The model under review builds one solid part; all positions refer to its coordinate system, in mm. Face numbers are marked on the shaded views. A direction names the side the tool comes from. Coordinates: 2 decimals unless noted, no trailing zeros. Write each loop counter-clockwise with the first axis right and the second up, starting at its lowest first coordinate (ties: lowest second). Pieces come first, ordered by that corner, then holes. Notation, with made-up numbers: (81.25, 25) - (131.25, 25) arc R26 cw to (131.25, 63) - close; hole circle Ø2 at (68, -30). An arc over 180 degrees is marked (long way). Put each result on its own line as item: value. Start each with the question number.
Item 1: For pin 1 (3 mm diameter, centred on x = -25.5, z = 3.5, fed in from +Y); pin 2 (5 mm diameter, centred on x = 12.5, z = 3, fed in from +Y); pin 3 (4 mm diameter, centred on x = -17, y = 5, fed in from +Z), all flat-tipped, find the tip position at first contact; note any pin that passes through.
Item 2: Consider section B-B on x = 3. Give the boundary of the cut face in (y, z), then the cut area to 3 significant figures.
Item 3: To check wall thickness, follow L1, parallel to Y at x = 7, z = 0; L2, parallel to X at y = -7.25, z = 4.5; L3, parallel to Y at x = 16, z = 0.75. State the ranges of each line that lie inside material, in increasing order. Write a range as [from, to].
Item 4: Machinability: for the marked faces 1 and 2, which of the approach directions +Z, -Z, +X, -X, +Y, -Y give a long, thin tool a straight path to every point of the face, cutting with its end or side? Answer none if there is none.
Item 5: Consider section C-C on x = 25.5. Give the boundary of the cut face in (y, z).
Item 6: Mouldability with a two-part tool opening along X and no side actions: class the marked faces 3, 4, 5 and 6 as pulls with the +X half, pulls with the -X half, needs draft (parallel to the pull), parting line crosses it, or undercut.
Item 7: Consider section A-A on x = 18.5. Give the boundary of the cut face in (y, z).
```python
from build123d import *

# Parameters (mm, degrees)
EXTRUDE1_DEPTH     = 6.08076
CIRPATTERN1_COUNT  = 2
CIRPATTERN1_ANGLE  = 90
SKETCH4_R          = 4.572
CUT_EXTRUDE1_DEPTH = 36.707811179


with BuildPart() as part:
    # Sketch1 → Revolve1 (revolve)
    with BuildSketch(Plane.XY, mode=Mode.PRIVATE) as revolve1_sk:
        Polygon((33.528, 4.572), (33.528, 5.715), (32.01924, 5.715), (21.45792, 7.239), (21.45792, 5.7912), (8.71728, 5.7912), (8.71728, 8.6868), (5.36448, 8.6868), (5.36448, 6.94944), (0, 6.94944), (0, 4.572), align=None)
    revolve(revolve1_sk.sketch.rotate(Axis((0, 0, 0), (1, 0, 0)), 90), axis=Axis((0, 0, 0), (1, 0, 0)))

    # Sketch2 → Revolve2 (revolve)
    with BuildSketch(Plane.XY, mode=Mode.PRIVATE) as revolve2_sk:
        with BuildLine():
            Line((11.61288, 5.7912), (8.71728, 5.7912))
            Line((8.71728, 5.7912), (8.71728, 8.6868))
            ThreePointArc((8.71728, 8.6868), (9.565381604, 6.639301604), (11.61288, 5.7912))
        make_face()
        with BuildLine():
            Line((5.36448, 8.6868), (5.36448, 6.94944))
            Line((5.36448, 6.94944), (3.62712, 6.94944))
            ThreePointArc((3.62712, 6.94944), (4.855619037, 7.458300963), (5.36448, 8.6868))
        make_face()
    revolve(revolve2_sk.sketch.rotate(Axis((0, 0, 0), (1, 0, 0)), 90), axis=Axis((0, 0, 0), (1, 0, 0)))

    # Sketch3 → Extrude1 (add, symmetric)
    with BuildSketch(Plane(origin=(0, 0, 0), x_dir=(-1, 0, 0), z_dir=(0, 0.7071067811865488, 0.7071067811865462))):
        with BuildLine():
            Line((-13.970508, 0.75438), (-19.100292, 0.75438))
            ThreePointArc((-19.100292, 0.75438), (-19.854672, 0), (-19.100292, -0.75438))
            Line((-19.100292, -0.75438), (-13.970508, -0.75438))
            ThreePointArc((-13.970508, -0.75438), (-13.216128, 0), (-13.970508, 0.75438))
        make_face()
    extrude1 = extrude(amount=EXTRUDE1_DEPTH, both=True)

    # CirPattern1: Extrude1 ×2 about axis
    cirpattern1_axis = Axis((0, 0, 0), (1, 0, 0))
    for i in range(1, CIRPATTERN1_COUNT):
        add(extrude1.rotate(cirpattern1_axis, i * CIRPATTERN1_ANGLE / (CIRPATTERN1_COUNT - 1)))

    # Sketch4 → Cut-Extrude1 (cut, through all)
    with BuildSketch(Plane(origin=(33.528, 0, 0), x_dir=(0, 0, -1), z_dir=(1, 0, 0))):
        with Locations(Location((0, 0, 0), (0, 0, 180))):
            Circle(SKETCH4_R)
    extrude(amount=-CUT_EXTRUDE1_DEPTH, mode=Mode.SUBTRACT)

    # Mirror1: part across plane


with BuildPart() as part_1:
    add(part.part)
    add(part.part.mirror(Plane(origin=(0, 0, 0), x_dir=(0, 0, 1), z_dir=(1, 0, 0))))


solid = part_1.part
```
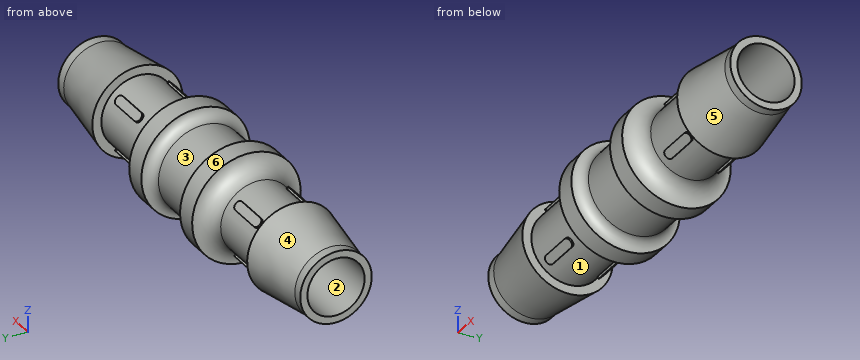
Report:
1. pin 1: y = 6.4
1. pin 2: y = 5.83
1. pin 3: z = 4.95
2. outline: circle Ø13.9 at (0, 0); hole circle Ø9.14 at (0, 0)
2. area: 86.1 mm²
3. L1: [-8.69, -4.57], [4.57, 8.69]
3. L2: [-8.72, -5.36], [5.36, 8.72]
3. L3: [-5.74, -4.51], [4.51, 5.74]
4. face 1: none
4. face 2: +X, -X
5. outline: circle Ø13.31 at (0, 0); hole circle Ø9.14 at (0, 0)
6. face 3: undercut
6. face 4: pulls with the -X half
6. face 5: pulls with the +X half
6. face 6: needs draft
7. outline: (-4.83, -3.77) - (-3.77, -4.83) - (-3.53, -4.59) arc R5.79 ccw to (3.53, -4.59) - (3.77, -4.83) - (4.83, -3.77) - (4.59, -3.53) arc R5.79 ccw to (4.59, 3.53) - (4.83, 3.77) - (3.77, 4.83) - (3.53, 4.59) arc R5.79 ccw to (-3.53, 4.59) - (-3.77, 4.83) - (-4.83, 3.77) - (-4.59, 3.53) arc R5.79 ccw to (-4.59, -3.53) - close; hole circle Ø9.14 at (0, 0)
